from build123d import *

# Parameters (mm, degrees)
SKETCH1_R                   = 2.5
SKETCH1_R_2                 = 3.25
BOSS_EXTRUDE1_DEPTH         = 2
TALADRO_ROSCADO_4_401_D     = 2.2606
TALADRO_ROSCADO_4_401_DEPTH = 12.7
TALADRO_ROSCADO_4_401_TIP   = 0.679152758


with BuildPart() as part:
    # Sketch1 → Boss-Extrude1 (new, symmetric)
    with BuildSketch(Plane.XY):
        with BuildLine():
            Line((0, -40), (0, 40))
            Line((0, 40), (-23.37, 40))
            ThreePointArc((-23.37, 40), (-27.223373178, 38.84392977), (-29.803954922, 35.757575758))
            Line((-29.803954922, 35.757575758), (-41.752728349, 7.878787879))
            ThreePointArc((-41.752728349, 7.878787879), (-43.37, 0), (-41.752728349, -7.878787879))
            Line((-41.752728349, -7.878787879), (-29.803954922, -35.757575758))
            ThreePointArc((-29.803954922, -35.757575758), (-27.223373178, -38.84392977), (-23.37, -40))
            Line((-23.37, -40), (0, -40))
        make_face()
        with Locations((-16.37, 30)):
            Circle(SKETCH1_R, mode=Mode.SUBTRACT)
        with Locations((-16.37, -30)):
            Circle(SKETCH1_R, mode=Mode.SUBTRACT)
        with Locations((-30.37, 0)):
            Circle(SKETCH1_R_2, mode=Mode.SUBTRACT)
    extrude(amount=BOSS_EXTRUDE1_DEPTH, both=True)

    # Taladro roscado #4-401
    with Locations(Plane.XY.offset(2)):
        with Locations((-30.37, -9.53), (-38.623222098, -4.765), (-38.623222098, 4.765), (-30.37, 9.53), (-22.116777902, 4.765), (-22.116777902, -4.765)):
            Hole(TALADRO_ROSCADO_4_401_D / 2, depth=TALADRO_ROSCADO_4_401_DEPTH)
            with Locations((0, 0, -(TALADRO_ROSCADO_4_401_DEPTH + TALADRO_ROSCADO_4_401_TIP / 2))):  # 118° drill point
                Cone(0, TALADRO_ROSCADO_4_401_D / 2, TALADRO_ROSCADO_4_401_TIP, mode=Mode.SUBTRACT)


solid = part.part
The listing builds one solid part. Answer for the finished solid, in the listing's coordinates (mm). Give positions to 0.01 mm unless a question says otherwise; leave off trailing zeros. Order: outer loops, then holes, each group sorted by start corner. A loop starts at its lowest first (then second) coordinate and runs counter-clockwise, first axis right, second up. Notation, with made-up numbers: (14, 8) - (62, 8) arc R9 ccw to (62, 15) - close; hole circle Ø1 at (3, 55.5). An arc over 180 degrees is marked (long way). Answer as CSV lines item,"result".
Q1. A cutting plane is placed at B-B, the plane z = 0.75. Count the separate pieces of the cut face and the enclosed holes in it, and give its area (3 significant figures).
Answer key:
separate pieces,"1"
enclosed holes,"9"
area,"2,810 mm^2"
Q2. Determine the mould class of faces 1 (the face through (-12, -40, 0)), 2 (the face through (-20.988, -4.715, -0.028)), 3 (the face through (-35.7, 22, 0)) for opening direction Y: pulls with the +Y half, pulls with the -Y half, needs draft (parallel to the pull), parting line crosses it, or undercut.
Answer key:
face 1,"pulls with the -Y half"
face 2,"undercut"
face 3,"pulls with the +Y half"
Q3. A cutting plane is placed at A-A, the plane y = 0. Determine the outline of the cut face in (x, z).
Answer key:
outline,"(-43.37, -2) - (-33.62, -2) - (-33.62, 2) - (-43.37, 2) - close; (-27.12, -2) - (0, -2) - (0, 2) - (-27.12, 2) - close"
Q4. A cutting plane is placed at C-C, the plane x = -18. Determine the outline of the cut face in (y, z), and give its area (3 significant figures).
Answer key:
outline,"(-40, -2) - (-31.9, -2) - (-31.9, 2) - (-40, 2) - close; (-28.1, -2) - (28.1, -2) - (28.1, 2) - (-28.1, 2) - close; (31.9, -2) - (40, -2) - (40, 2) - (31.9, 2) - close"
area,"290 mm^2"
Q5. A cutting plane is placed at D-D, the plane y = -28.5. Determine the outline of the cut face in (x, z).
Answer key:
outline,"(-32.91, -2) - (-18.37, -2) - (-18.37, 2) - (-32.91, 2) - close; (-14.37, -2) - (0, -2) - (0, 2) - (-14.37, 2) - close"
Q6. Straight lines are drawn through the part: L1, parallel to Y at x = -18.5, z = -1.7; L2, parallel to Y at x = -38, z = 1.8; L3, parallel to Y at x = -30.37, z = -0.85. For each, find the intervals that lie inside material, in ascending order.
Answer key:
L1,"y = -40 to -31.31, -28.69 to 28.69, 31.31 to 40"
L2,"y = -16.63 to -5.71, -3.82 to 3.82, 5.71 to 16.63"
L3,"y = -34.44 to -10.66, -8.4 to -3.25, 3.25 to 8.4, 10.66 to 34.44"
Q7. This flat-tipped pin is pushed along its axis until it touches: pin 1 Ø2 at (y, z) = (24.5, 0.5) entering from -X. Where does it stop, or does it pass through?
Answer key:
pin 1,"stops at x = -35.06"
